Autodesk Fusion 360 part; units mm, degrees
sketch "Sketch1" plane through (0, 0, 0) normal (1, 0, 0) x (0, 1, 0)
  line L0 (-48, 0) -> (-51, 0)
  line L1 (-48, 0) -> (-51, 0)
  line L2 (48, 0) -> (51, 0)
  line L3 (-51, 0) -> (-51, 40.2989)
  line L4 (51, 0) -> (51, 40.2989)
  arc A0 (48, 36) -> (-48, 36) centre (0, 0) ccw
  arc A1 (51, 40.2989) -> (-51, 40.2989) centre (0, 0) ccw
  line L5 (-51, 0) -> (-48, 0)
  line L6 (-48, 15) -> (-48, 36)
  line L7 (-48, 15) -> (-48, 0)
  line L8 (48, 20.1494) -> (48, 36)
  line L9 (48, 20.1494) -> (48, 0)
  dimension "d1" = 51
  dimension "d2" = 51
  dimension "d3" = 130
extrude "Extrude1" add sketch "Sketch1" along normal blind 105
hole "Hole1" at (61.1241, 0, 65) direction (0, 0, -1) diameter 3 depth 10 tip angle 118
hole "Hole2" at (38.2805, 0, 65) direction (0, 0, -1) diameter 3 depth 10 tip angle 118
Work out the finished part from the listing and answer in its coordinate system (mm). A direction names the side the tool comes from. Coordinates: 2 decimals unless noted, no trailing zeros. Write each loop counter-clockwise with the first axis right and the second up, starting at its lowest first coordinate (ties: lowest second). Pieces come first, ordered by that corner, then holes.
Q1. A cutting plane is placed at C-C, the plane z = 45. Give the vertices of the cut face in (x, y), then the cut area to 3 significant figures.
Q2. Find the intervals of material crossed by line 1 (X direction, y = 0, z = 63.4); line 2 (Y direction, x = 100.5, z = 7); line 3 (Y direction, x = 15, z = 40), in increasing order.
Q3. A cutting plane is placed at D-D, the plane y = 11. Give the vertices of the cut face in (x, z).
Q4. Determine the mould class of faces 3 (the face through (0, 0, 62)), 4 (the face through (52, 51, 20)), 5 (the face through (52, 48, 18)), 6 (the face through (51.765, -0.821, 64.995)) for opening direction Y: released by +Y, released by -Y, zero draft, split by the parting line, or undercut.
Q5. Which of the six approach directions +Z, -Z, +X, -X, +Y, -Y give full straight-line access (tool end or side, diameter ignored) to faces 1 (the face through (39.193, 1.19, 62.455)), 2 (the face through (52, -48, 18))?
Q6. A cutting plane is placed at A-A, the plane z = 7. Give the vertices of the cut face in (x, y), then the cut area to 3 significant figures.
Q7. Each of these flat-tipped pins is pushed along its axis until it touches: pin 1 Ø6 at (x, y) = (44, -2) entering from -Z; pin 2 Ø12 at (x, y) = (30, 18) entering from +Z; pin 3 Ø1 at (x, y) = (77, 15) entering from +Z. Where does it stop, or does it pass through?
Q8. A cutting plane is placed at B-B, the plane x = 71. Give the vertices of the cut face in (y, z), then the cut area to 3 significant figures.
Findings below:
1. outline: (0, -46.9) - (105, -46.9) - (105, -39.69) - (0, -39.69) - close; (0, 39.69) - (105, 39.69) - (105, 46.9) - (0, 46.9) - close
1. area: 1,520 mm2
2. line 1: x = 0 to 36.78, 39.78 to 59.62, 62.62 to 105
2. line 2: y = -51 to -48, 48 to 51
2. line 3: y = -51 to -44.72, 44.72 to 51
3. outline: (0, 58.98) - (105, 58.98) - (105, 64.06) - (0, 64.06) - close
4. face 3: zero draft
4. face 4: released by +Y
4. face 5: undercut
4. face 6: split by the parting line
5. face 1: +Z, -Z
5. face 2: -Z, +X, -X
6. outline: (0, -51) - (105, -51) - (105, -48) - (0, -48) - close; (0, 48) - (105, 48) - (105, 51) - (0, 51) - close
6. area: 630 mm2
7. pin 1: stops at z = 59.79
7. pin 2: stops at z = 63.88
7. pin 3: stops at z = 63.36
8. outline: (-51, 0) - (-48, 0) - (-48, 36) arc R60 cw to (48, 36) - (48, 0) - (51, 0) - (51, 40.3) arc R65 ccw to (-51, 40.3) - close
8. area: 800 mm2
